Work out the finished part from the listing and answer in its coordinate system (mm). Round coordinates to 2 decimals unless told otherwise and drop trailing zeros. Loops run counter-clockwise (first coordinate to the right, second up) from the corner with the lowest first, then second, coordinate; pieces in that order, holes last.
```python
from build123d import *

# Parameters (mm, degrees)
F0_W     = 445
F0_H     = 445
F1_DEPTH = 18
F2_R     = 2.5
F3_DEPTH = 15
F4_R     = 3.5
F5_DEPTH = 70


# Not quite as in the source:
# - a pattern or mirror of a feature is missing from the dataset's text; its kind, count and spacing are read off the source's solid


with BuildPart() as f1:
    # F0 (on Front) → F1 (new body)
    with BuildSketch(Plane.XZ):
        Rectangle(F0_W, F0_H)
    extrude(amount=F1_DEPTH)

    # F2 (on face) → F3 (join)
    with BuildSketch(Plane.XZ.offset(18)):
        with Locations((-172.5, 50)):
            Circle(F2_R)
    f3 = extrude(amount=F3_DEPTH)

    # F3_copies: F3 across plane
    add(f3.mirror(Plane(origin=(0, 0, -1e-05), x_dir=(-1, 0, 0), z_dir=(0, 0, -1))))

    # F4 (on Top) → F5 (join, symmetric)
    with BuildSketch(Plane.XY):
        with Locations((-172.5, -33)):
            Circle(F4_R)
    extrude(amount=F5_DEPTH, both=True)


solid = f1.part
```
1. Find section A-A (z = -10.5). Write down the section's boundary in (x, y).
Answer key:
outline: (-222.5, -18) - (222.5, -18) - (222.5, 0) - (-222.5, 0) - close; circle Ø7 at (-172.5, -33)
2. Given pin 1 (2 mm diameter, centred on x = -171.5, y = -32, fed in from -Z); pin 2 (5 mm diameter, centred on y = -29.5, z = -67, fed in from +X); pin 3 (2 mm diameter, centred on x = -171, y = -32, fed in from +Z), each flat-ended and moving along its own axis, determine where each tip first touches the part or whether it passes through.
Answer key:
pin 1: stops at z = -70
pin 2: stops at x = -169.15
pin 3: stops at z = 70
3. Find section B-B (z = -108.5). Write down the section's boundary in (x, y), then the cut area to 3 significant figures.
Answer key:
outline: (-222.5, -18) - (222.5, -18) - (222.5, 0) - (-222.5, 0) - close
area: 8,010 mm2
4. Find section C-C (x = -117.5). Write down the section's boundary in (y, z), then the cut area to 3 significant figures.
Answer key:
outline: (-18, -222.5) - (0, -222.5) - (0, 222.5) - (-18, 222.5) - close
area: 8,010 mm2
5. Consider probe 1 along Y at (x, z) = (179, 58). Determine where the line is inside the solid, lowest interval first.
Answer key:
probe 1: y = -18 to 0
